Work out the finished part from the listing and answer in its coordinate system (mm). A direction names the side the tool comes from. Round coordinates to 2 decimals unless told otherwise and drop trailing zeros. Write each loop counter-clockwise with the first axis right and the second up, starting at its lowest first coordinate (ties: lowest second). Pieces come first, ordered by that corner, then holes. Notation, with made-up numbers: (43, 24) - (72, 24) arc R18 ccw to (72, 44) - close; hole circle Ø2 at (61, 60). An arc over 180 degrees is marked (long way). Answer as a JSON object with one key per item and string values.
```python
from build123d import *

# Parameters (mm, degrees)
F1_DEPTH = 25
F3_D     = 5.5
F3_DEPTH = 12
F3_TIP   = 1.6523667023


with BuildPart() as f1:
    # F0 (on Top) → F1 (new body)
    with BuildSketch(Plane.XY):
        with BuildLine():
            Line((20, 35.7499521262), (-60, 35.7499521262))
            ThreePointArc((-60, 35.7499521262), (-63.5355339059, 34.2854860321), (-65, 30.7499521262))
            Line((-65, 30.7499521262), (-65, 0))
            Line((-65, 0), (0, 0))
            Line((0, 0), (0, -24.2500478738))
            Line((0, -24.2500478738), (20, -24.2500478738))
            Line((20, -24.2500478738), (20, 35.7499521262))
        make_face()
    extrude(amount=F1_DEPTH)

    # F3
    with Locations(Plane.XY.offset(25)):
        with Locations((-15, 20.7499521262)):
            Hole(F3_D / 2, depth=F3_DEPTH)
            with Locations((0, 0, -(F3_DEPTH + F3_TIP / 2))):  # 118° drill point
                Cone(0, F3_D / 2, F3_TIP, mode=Mode.SUBTRACT)


solid = f1.part
```
Item 1: A cutting plane is placed at B-B (x = -19). Write down the section's boundary in (y, z), and give its area (3 significant figures).
Results found:
{"outline": "(0, 0) - (35.75, 0) - (35.75, 25) - (0, 25) - close", "area": "894 mm²"}
Item 2: A cutting plane is placed at D-D (y = -12.5). Write down the section's boundary in (x, z), and give its area (3 significant figures).
Results found:
{"outline": "(0, 0) - (20, 0) - (20, 25) - (0, 25) - close", "area": "500 mm²"}
Item 3: For faces 1 (the flat face through (0, -12, 12)), 2 (the flat face through (-65, 16, 12)), determine the directions among +Z, -Z, +X, -X, +Y, -Y from which every point of the face is accessible in a straight line to the end or side of a thin tool.
Results found:
{"face 1": "+Z, -Z, -X, -Y", "face 2": "+Z, -Z, -X, +Y, -Y"}
Item 4: Determine the mould class of faces 3 (the flat face through (-19, 35.75, 12)), 4 (the flat face through (-33, 0, 12)), 5 (the flat face through (-14, 13, 0)), 6 (the cylindrical face through (-14.642, 23.477, 18.916)) for opening direction Y: pulls with the +Y half, pulls with the -Y half, needs draft (parallel to the pull), parting line crosses it, or undercut.
Results found:
{"face 3": "pulls with the +Y half", "face 4": "pulls with the -Y half", "face 5": "needs draft", "face 6": "undercut"}
Item 5: Consider line 1 along Y through (x, z) = (-15, 15.75); line 2 along Y through (x, z) = (-24.5, 14.75); line 3 along X through (y, z) = (-17, 21.25). Determine where each line is inside the solid, lowest interval first.
Results found:
{"line 1": "0 to 18, 23.5 to 35.75", "line 2": "0 to 35.75", "line 3": "0 to 20"}
Item 6: A cutting plane is placed at A-A (z = 10). Write down the section's boundary in (x, y).
Results found:
{"outline": "(-65, 0) - (0, 0) - (0, -24.25) - (20, -24.25) - (20, 35.75) - (-60, 35.75) arc R5 ccw to (-65, 30.75) - close"}
Item 7: A cutting plane is placed at C-C (z = 20.75). Write down the section's boundary in (x, y), and give its area (3 significant figures).
Results found:
{"outline": "(-65, 0) - (0, 0) - (0, -24.25) - (20, -24.25) - (20, 35.75) - (-60, 35.75) arc R5 ccw to (-65, 30.75) - close; hole circle Ø5.5 at (-15, 20.75)", "area": "3,490 mm²"}
Item 8: Each of these flat-tipped pins is pushed along its axis until it touches: P1, Ø4.5, axis at x = -15, y = 20.75, coming from the +Z side; P2, Ø7.5, axis at y = -8, z = 18.5, coming from the -X side. Where does it stop, or does it pass through?
Results found:
{"P1": "z = 12.7", "P2": "x = 0"}
